Design review of the part shown in the three views and the two pictorial views. Dimensions are in mm from the part's minimum x, y and z. A direction names the side the tool comes from. Round coordinates to 2 decimals unless told otherwise and drop trailing zeros. Return JSON: item names as keys, results as strings. Group by question number.
1. Clearance check with flat-ended pins moving along their axes: P1, Ø6, axis at x = 12.5, y = 10, coming from the +Z side (1 decimal); P2, Ø1.5, axis at y = 11, z = 7, coming from the -X side (1 decimal). State where each tip first meets the part, or that it passes through.
2. Tool access review of the marked faces 4 and 5: name each direction out of +Z, -Z, +X, -X, +Y, -Y from which nothing blocks a thin tool from reaching the whole face with its end or side.
3. For line 1 along Z through (x, y) = (15.25, 11.75) (1 decimal); line 2 along Y through (x, z) = (18, 9), list the stretches that pass through material, from the lowest coordinate up. Write a range as from..to.
4. Mouldability with a two-part tool opening along Z and no side actions: class the marked faces 1, 2 and 3 as pulls with the +Z half, pulls with the -Z half, needs draft (parallel to the pull), parting line crosses it, or undercut.
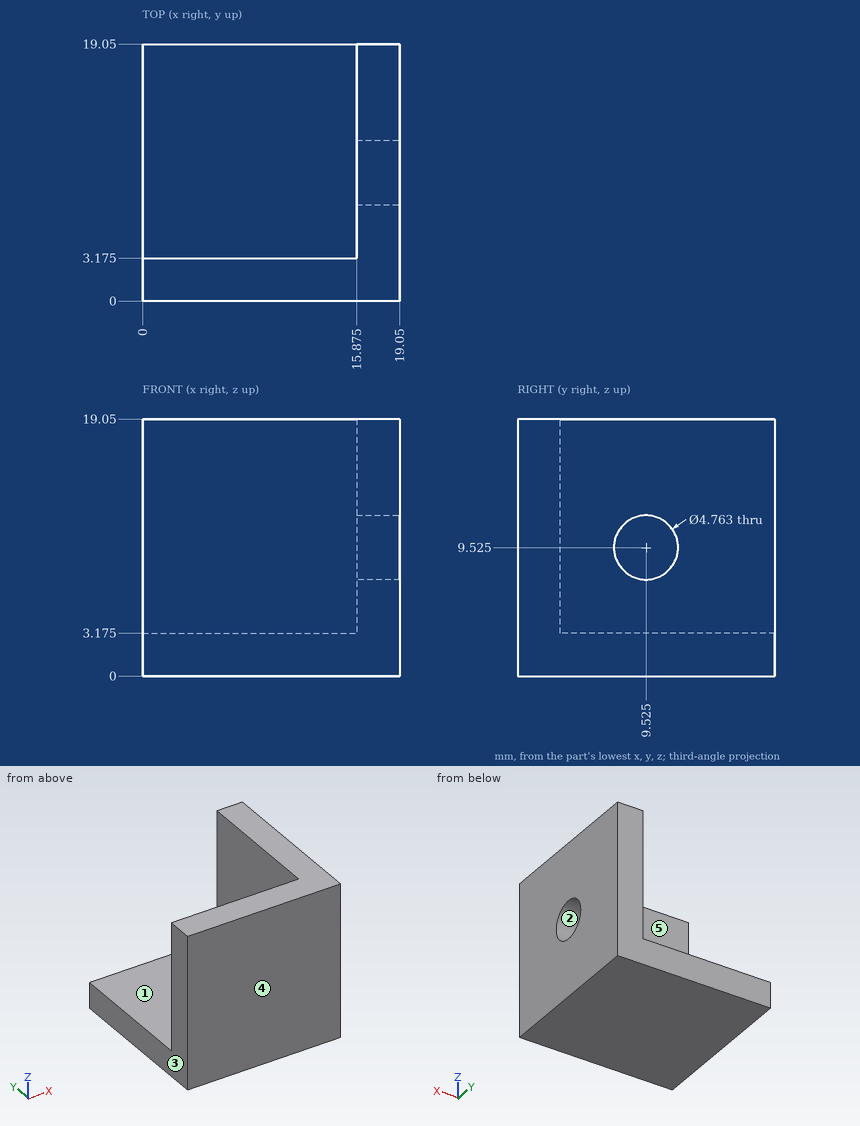
Output:
{
 "1": {"P1": "stops at z = 3.2", "P2": "stops at x = 15.9"},
 "2": {"face 4": "+Z, -Z, +X, -X, -Y", "face 5": "+Z, -X, +Y"},
 "3": {"line 1": "z = 0..3.2", "line 2": "y = 0..7.2, 11.85..19.05"},
 "4": {"face 1": "pulls with the +Z half", "face 2": "undercut", "face 3": "needs draft"}
}
